For this review, take the finished solid that the model builds, in its own axes (mm). Round coordinates to 2 decimals unless told otherwise and drop trailing zeros. Order: outer loops, then holes, each group sorted by start corner. A loop starts at its lowest first (then second) coordinate and runs counter-clockwise, first axis right, second up. Notation, with made-up numbers: M 29,70.25 L 33,70.25 A24 ccw 33,98.25 Z; hole C 54,-9 d9. An arc over 180 degrees is marked long. Answer as a JSON object with one key per item and string values.
from build123d import *

# Parameters (mm, degrees)
BOSS_EXTRUDE1_DEPTH = 6.35
SKETCH2_R           = 1.35
SKETCH2_R_2         = 1.385
CUT_EXTRUDE1_DEPTH  = 38.116505762
SKETCH3_W           = 63.5
SKETCH3_H           = 71.12
SKETCH3_W_2         = 38.321076004
SKETCH3_H_2         = 47.237540142
BOSS_EXTRUDE2_DEPTH = 6.35
SKETCH5_W           = 27.94
SKETCH5_H           = 55.88
CUT_EXTRUDE3_DEPTH  = 51.07984184
SKETCH7_W           = 69.85
SKETCH7_H           = 0.368341575
CUT_EXTRUDE4_DEPTH  = 10
SKETCH9_R           = 2
CUT_EXTRUDE5_DEPTH  = 51.07984184
SKETCH10_W          = 41.322373354
SKETCH10_H          = 59.668082212
BOSS_EXTRUDE3_DEPTH = 6.35
SKETCH11_R          = 6
CUT_EXTRUDE6_DEPTH  = 51.07984184
FILLET1_R           = 5.08
FILLET2_R           = 5.08
FILLET3_R           = 5.08


with BuildPart() as part:
    # Sketch1 → Boss-Extrude1 (new body)
    with BuildSketch(Plane.XY):
        with BuildLine():
            Line((-19.69889026, 23.2987845), (-14.850045261, 29.75147823))
            ThreePointArc((-14.850045261, 29.75147823), (-14.144755454, 30.339267512), (-13.251155001, 30.55))
            Line((-13.251155001, 30.55), (13.251155001, 30.55))
            ThreePointArc((13.251155001, 30.55), (14.144755454, 30.339267512), (14.850045261, 29.75147823))
            Line((14.850045261, 29.75147823), (19.69889026, 23.2987845))
            ThreePointArc((19.69889026, 23.2987845), (19.997074131, 22.730638521), (20.1, 22.09730627))
            Line((20.1, 22.09730627), (20.1, -22.09730627))
            ThreePointArc((20.1, -22.09730627), (19.997074131, -22.730638521), (19.69889026, -23.2987845))
            Line((19.69889026, -23.2987845), (14.850045261, -29.75147823))
            ThreePointArc((14.850045261, -29.75147823), (14.144755454, -30.339267512), (13.251155001, -30.55))
            Line((13.251155001, -30.55), (-13.251155001, -30.55))
            ThreePointArc((-13.251155001, -30.55), (-14.144755454, -30.339267512), (-14.850045261, -29.75147823))
            Line((-14.850045261, -29.75147823), (-19.69889026, -23.2987845))
            ThreePointArc((-19.69889026, -23.2987845), (-19.997074131, -22.730638521), (-20.1, -22.09730627))
            Line((-20.1, -22.09730627), (-20.1, 22.09730627))
            ThreePointArc((-20.1, 22.09730627), (-19.997074131, 22.730638521), (-19.69889026, 23.2987845))
        make_face()
    extrude(amount=-BOSS_EXTRUDE1_DEPTH)

    # Sketch2 → Cut-Extrude1 (cut, through all)
    with BuildSketch(Plane(origin=(0, 0, -6.35), x_dir=(-1, 0, 0), z_dir=(0, 0, -1))):
        with Locations((17.3, 21.9487845)):
            Circle(SKETCH2_R)
        with Locations((17.3, -0.0512155)):
            Circle(SKETCH2_R)
        with Locations((17.3, -22.0512155)):
            Circle(SKETCH2_R)
        with Locations((11, -27.75)):
            Circle(SKETCH2_R_2)
        with Locations(Location((-11, -27.75, 0), (0, 0, 180))):
            Circle(SKETCH2_R_2)
        with Locations(Location((-17.3, -22.0512155, 0), (0, 0, 180))):
            Circle(SKETCH2_R)
        with Locations(Location((-17.3, -0.0512155, 0), (0, 0, 180))):
            Circle(SKETCH2_R)
        with Locations(Location((-17.3, 21.9487845, 0), (0, 0, 180))):
            Circle(SKETCH2_R)
    extrude(amount=-CUT_EXTRUDE1_DEPTH, mode=Mode.SUBTRACT)

    # Sketch3 → Boss-Extrude2 (add)
    with BuildSketch(Plane(origin=(0, 0, -6.35), x_dir=(-1, 0, 0), z_dir=(0, 0, -1))):
        with Locations((0, 2.6447845)):
            Rectangle(SKETCH3_W, SKETCH3_H)
        Rectangle(SKETCH3_W_2, SKETCH3_H_2, mode=Mode.SUBTRACT)
    extrude(amount=-BOSS_EXTRUDE2_DEPTH)

    # Sketch5 → Cut-Extrude3 (cut, through all)
    with BuildSketch(Plane.XY):
        with Locations((0, 3.0087845)):
            Rectangle(SKETCH5_W, SKETCH5_H)
    extrude(amount=-CUT_EXTRUDE3_DEPTH, mode=Mode.SUBTRACT)

    # Sketch7 → Cut-Extrude4 (cut)
    with BuildSketch(Plane.XY):
        with Locations((3.175, -32.731044713)):
            Rectangle(SKETCH7_W, SKETCH7_H)
    extrude(amount=-CUT_EXTRUDE4_DEPTH, mode=Mode.SUBTRACT)

    # Sketch9 → Cut-Extrude5 (cut, through all)
    with BuildSketch(Plane.XY):
        with Locations((25.4, 31.8547845)):
            Circle(SKETCH9_R)
        with Locations((-25.4, 31.8547845)):
            Circle(SKETCH9_R)
        with Locations((-25.4, -26.196873925)):
            Circle(SKETCH9_R)
        with Locations((25.4, -26.196873925)):
            Circle(SKETCH9_R)
    extrude(amount=-CUT_EXTRUDE5_DEPTH, mode=Mode.SUBTRACT)

    # Sketch10 → Boss-Extrude3 (add)
    with BuildSketch(Plane(origin=(0, 0, -6.35), x_dir=(-1, 0, 0), z_dir=(0, 0, -1))):
        with Locations((0, 2.205557414)):
            Rectangle(SKETCH10_W, SKETCH10_H)
    extrude(amount=-BOSS_EXTRUDE3_DEPTH)

    # Sketch11 → Cut-Extrude6 (cut, through all)
    with BuildSketch(Plane.XY):
        with Locations((0, 17.8847845)):
            Circle(SKETCH11_R)
    extrude(amount=-CUT_EXTRUDE6_DEPTH, mode=Mode.SUBTRACT)

    # Fillet1
    fillet1_edges = [part.edges().sort_by_distance(p)[0] for p in [
        (-31.75, 38.2047845, -3.175),
    ]]
    fillet(fillet1_edges, radius=FILLET1_R)

    # Fillet2
    fillet2_edges = [part.edges().sort_by_distance(p)[0] for p in [
        (31.75, -32.546873925, -3.175),
        (31.75, 38.2047845, -3.175),
    ]]
    fillet(fillet2_edges, radius=FILLET2_R)

    # Fillet3
    fillet3_edges = [part.edges().sort_by_distance(p)[0] for p in [
        (-31.75, -32.546873925, -3.175),
    ]]
    fillet(fillet3_edges, radius=FILLET3_R)


solid = part.part
1) Add section D-D on z = -1.75. State the section outline as (x, y) points.
Geometry check:
{"outline": "M -31.75,-27.47 A5.08 ccw -26.67,-32.55 L 26.67,-32.55 A5.08 ccw 31.75,-27.47 L 31.75,33.12 A5.08 ccw 26.67,38.2 L -26.67,38.2 A5.08 ccw -31.75,33.12 Z; hole C -25.4,-26.2 d4; hole C -25.4,31.85 d4; hole C 0,17.88 d12; hole C 25.4,-26.2 d4; hole C 25.4,31.85 d4"}
2) Add section A-A on x = 0. State the section outline as (y, z) points.
Geometry check:
{"outline": "M -32.55,-6.35 L 11.88,-6.35 L 11.88,0 L -32.55,0 Z; M 23.88,-6.35 L 38.2,-6.35 L 38.2,0 L 23.88,0 Z"}
3) For L1, parallel to Y at x = -25.4, z = -1.5; L2, parallel to X at y = 32, z = -5.5; L3, parallel to Y at x = 26.5, z = -4, list the stretches that pass through material, from the lowest coordinate up.
Geometry check:
{"L1": "y = -32.55 to -28.2, -24.2 to 29.85, 33.85 to 38.2", "L2": "x = -31.75 to -27.39, -23.41 to 23.41, 27.39 to 31.75", "L3": "y = -32.55 to -27.87, -24.53 to 30.18, 33.53 to 38.2"}
4) Insertion check: P1, Ø12, axis at x = 13, y = -1.5, coming from the +Z side. The pin has a flat end and moves straight along its axis. Give the tip position at first contact, or say it passes through.
Geometry check:
{"P1": "stops at z = 0"}
5) Add section C-C on y = 16. State the section outline as (x, z) points, and give its area (3 significant figures).
Geometry check:
{"outline": "M -31.75,-6.35 L -5.7,-6.35 L -5.7,0 L -31.75,0 Z; M 5.7,-6.35 L 31.75,-6.35 L 31.75,0 L 5.7,0 Z", "area": "331 mm²"}
6) Add section B-B on x = -25.4. State the section outline as (y, z) points, and give its area (3 significant figures).
Geometry check:
{"outline": "M -32.55,-6.35 L -28.2,-6.35 L -28.2,0 L -32.55,0 Z; M -24.2,-6.35 L 29.85,-6.35 L 29.85,0 L -24.2,0 Z; M 33.85,-6.35 L 38.2,-6.35 L 38.2,0 L 33.85,0 Z", "area": "398 mm²"}
7) Mouldability with a two-part tool opening along X and no side actions: class faces 1 (the cylindrical face through (27.31, -25.6, -3.13)), 2 (the cylindrical face through (30.3, -31.02, -3.13)), 3 (the flat face through (0, 38.205, -3)) as +X half, -X half, draft (parallel to the pull), parting line (faces both ways), or undercut.
Geometry check:
{"face 1": "undercut", "face 2": "+X half", "face 3": "draft"}
